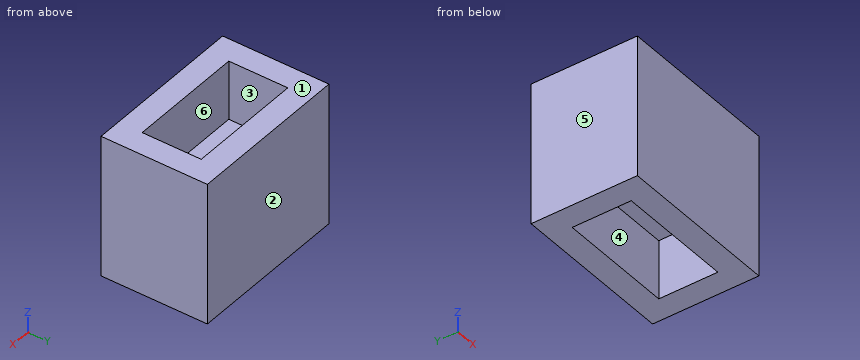
Autodesk Inventor part; units mm, degrees
ref_plane "YZ Plane" through (0, 0, 0) normal (1, 0, 0) x (0, 1, 0)
ref_plane "XZ Plane" through (0, 0, 0) normal (0, 1, 0) x (-1, 0, 0)
ref_plane "XY Plane" through (0, 0, 0) normal (0, 0, 1) x (1, 0, 0)
sketch "Sketch5" plane through (0, 0, 0) normal (0, 0, 1) x (1, 0, 0)
  line L0 (0, 0) -> (-13.9, 0)
  line L1 (-13.9, 0) -> (-13.9, 9)
  line L2 (-13.9, 9) -> (0, 9)
  line L3 (0, 9) -> (0, 0)
  line L4 (-2, 2) -> (-11.9, 2)
  line L5 (-11.9, 2) -> (-11.9, 7)
  line L6 (-11.9, 7) -> (-2, 7)
  line L7 (-2, 7) -> (-2, 2)
  dimension "d67" = 13.9
  dimension "d68" = 9
  dimension "d69" = 9.9
  dimension "d70" = 5
extrude "Extrusion8" add sketch "Sketch5" along normal blind 12 contours L0 L1 L2 L3 | L4 L5 L6 L7
sketch "Sketch6" plane through (0, 0, 12) normal (0, 0, 1) x (1, 0, 0)
  line L0 (-2, 2) -> (-11.9, 2)
  line L1 (-11.9, 2) -> (-11.9, 7)
  line L2 (-11.9, 7) -> (-2, 7)
  line L3 (-2, 7) -> (-2, 2)
  point P0 (0, 0)
  dimension "d73" = 9.9
  dimension "d74" = 5
extrude "Extrusion9" cut sketch "Sketch6" against normal blind 5
sketch "Sketch7" plane through (0, 0, 0) normal (0, 0, -1) x (-1, 0, 0)
  line L0 (2, 2) -> (11.9, 2)
  line L1 (11.9, 2) -> (11.9, 7)
  line L2 (11.9, 7) -> (2, 7)
  line L3 (2, 7) -> (2, 2)
  point P0 (0, 0)
  dimension "d77" = 9.9
  dimension "d78" = 5
extrude "Extrusion11" cut sketch "Sketch7" against normal blind 5
properties part number "Cube_Holder_SB_V1_(71mm)"
Check sheet for the modelled part. Datum: model origin and axes. Units: mm. Face numbers are marked on the shaded views. A direction names the side the tool comes from. Round coordinates to 2 decimals unless told otherwise and drop trailing zeros. Write each loop counter-clockwise with the first axis right and the second up, starting at its lowest first coordinate (ties: lowest second). Pieces come first, ordered by that corner, then holes. Notation, with made-up numbers: (45.5, 49.25) -> (97.5, 49.25) arc R17 cw to (97.5, 81.25) -> close; hole circle Ø11 at (75, -0.75). An arc over 180 degrees is marked (long way). Put each result on its own line as item: value.
(1) Sectioned sample at A-A (z = 4). Enter the section's corners in (x, y).
Values found:
outline: (-13.9, 0) -> (0, 0) -> (0, 9) -> (-13.9, 9) -> close; hole (-11.9, 2) -> (-2, 2) -> (-2, 7) -> (-11.9, 7) -> close
(2) Mould release check, pull along Y, two halves, no side actions. Record for the marked faces 1, 2 and 3: released by +Y, released by -Y, zero draft, split by the parting line, or undercut.
Values found:
face 1: zero draft
face 2: released by +Y
face 3: undercut
(3) Tool access check on the marked faces 4, 5 and 6. Record the directions out of +Z, -Z, +X, -X, +Y, -Y that give a thin tool (end or side, any length) a straight path to the whole face; none if there is none.
Values found:
face 4: -Z
face 5: +Z, -Z, -X, +Y, -Y
face 6: +Z
(4) Material ranges on line 1 (X direction, y = 4.75, z = 0.5); line 2 (Y direction, x = -6, z = 11.25); line 3 (Z direction, x = -8.5, y = 6), recorded low to high.
Values found:
line 1: x = -13.9 to -11.9, -2 to 0
line 2: y = 0 to 2, 7 to 9
line 3: z = 5 to 7
(5) Sectioned sample at C-C (y = 3.75). Enter the section's corners in (x, z), plus the area to 3 significant figures.
Values found:
outline: (-13.9, 0) -> (-11.9, 0) -> (-11.9, 5) -> (-2, 5) -> (-2, 0) -> (0, 0) -> (0, 12) -> (-2, 12) -> (-2, 7) -> (-11.9, 7) -> (-11.9, 12) -> (-13.9, 12) -> close
area: 67.8 mm^2
(6) Go/stop test with a flat-tipped pin: pin 1 Ø1.5 at (x, y) = (-4.5, 5.5) entering from -Z. Record where the tip stops, or that it passes through.
Values found:
pin 1: stops at z = 5
(7) Sectioned sample at B-B (x = -8.5). Enter the section's corners in (y, z).
Values found:
outline: (0, 0) -> (2, 0) -> (2, 5) -> (7, 5) -> (7, 0) -> (9, 0) -> (9, 12) -> (7, 12) -> (7, 7) -> (2, 7) -> (2, 12) -> (0, 12) -> close
